Here's how the part is built. I have some questions about the finished solid (model axes, mm). Give positions to 0.01 mm unless a question says otherwise; leave off trailing zeros. Loops run counter-clockwise (first coordinate to the right, second up) from the corner with the lowest first, then second, coordinate; pieces in that order, holes last.
Q1. I need wall thicknesses on line 1 (Z direction, x = -6.5, y = 2.5); line 2 (Z direction, x = -11.5, y = 4.5); line 3 (Z direction, x = 27, y = 2.2). Which ranges of each line are inside material? Lowest first, please.
Q2. If we section it at B-B (z = 39.5): Please give me the cut outline in (x, y), plus the area to 3 significant figures.
Q3. If we section it at C-C (y = 1.4): Give the number of separate pieces and of enclosed holes in the cut face, plus the area to 3 significant figures.
Q4. If we section it at A-A (z = 81): Please give me the cut outline in (x, y), plus the area to 3 significant figures.
Q5. Will these pins go through, and if not, where does the flat tip stop? P1, Ø1.5, axis at y = 2.5, z = -119, coming from the +X side; P2, Ø1.5, axis at x = -4.5, y = 3, coming from the -Z side; P3, Ø8, axis at x = -21, z = 39.5, coming from the +Y side (3 decimals).
from build123d import *

# Parameters (mm, degrees)
BOSS_EXTRUDE1_DEPTH = 5
CHAMFER1_SIZE       = 10
SKETCH2_W           = 52.240142394
SKETCH2_H           = 49.910170897
SKETCH2_H_2         = 19.468376047
CUT_EXTRUDE1_DEPTH  = 5
CHAMFER2_SIZE       = 10


# Some blends are built 0.0001 mm under size
with BuildPart() as part:
    # Sketch1 → Boss-Extrude1 (new body)
    with BuildSketch(Plane(origin=(0, 0, 0), x_dir=(1, 0, 0), z_dir=(0, 1, 0))):
        Polygon((12.5, 112.5), (40, 112.5), (40, -112.5), (-40, -112.5), (-40, 112.5), (-12.5, 112.5), (-12.5, 122.5), (-8, 122.5), (-8, 112.5), (8, 112.5), (8, 122.5), (12.5, 122.5), align=None)
        Polygon((35, -71.386750493), (35, -77.596695784), (35.5, -77.596695784), (35.5, -90.016586366), (-35.5, -90.016586366), (-35.5, -77.596695784), (-35, -77.596695784), (-35, -71.386750493), align=None, mode=Mode.SUBTRACT)
    extrude(amount=BOSS_EXTRUDE1_DEPTH)

    # Chamfer1
    chamfer1_edges = [part.edges().sort_by_distance(p)[0] for p in [
        (-12.5, 2.5, -112.5),
        (12.5, 2.5, -112.5),
    ]]
    chamfer(chamfer1_edges, length=CHAMFER1_SIZE - 0.0001)  # a hair under: the kernel refuses the full size

    # Sketch2 → Cut-Extrude1 (cut)
    with BuildSketch(Plane(origin=(0, 5, 0), x_dir=(1, 0, 0), z_dir=(0, 1, 0))):
        with Locations((0, 36.827678023)):
            Rectangle(SKETCH2_W, SKETCH2_H)
        with Locations((0, -36.827678023)):
            Rectangle(SKETCH2_W, SKETCH2_H)
        with Locations((0, 81.251139518)):
            Rectangle(SKETCH2_W, SKETCH2_H_2)
    extrude(amount=-CUT_EXTRUDE1_DEPTH, mode=Mode.SUBTRACT)

    # Chamfer2
    # the kernel refuses this chamfer: 10 mm, written as the material it adds along each edge
    with BuildSketch(Plane(origin=(26.120071197, 5, -90.985327541), x_dir=(-0.9996219169112968, 0, -0.027495876610586317), z_dir=(0, -1, 0)), Plane(origin=(26.120071197, 5, -71.516951494), x_dir=(0.027495876610586317, 0, -0.9996219169112968), z_dir=(0, -1, 0)), Plane(origin=(-26.120071197, 5, -71.516951494), x_dir=(0.9996219169112968, 0, 0.027495876610586317), z_dir=(0, -1, 0)), Plane(origin=(-26.120071197, 5, 11.872592574), x_dir=(-0.027495876610586667, 0, 0.9996219169112968), z_dir=(0, -1, 0)), Plane(origin=(26.120071197, 5, 11.872592574), x_dir=(-0.9996219169112968, 0, -0.027495876610586317), z_dir=(0, -1, 0)), Plane(origin=(26.120071197, 5, 61.782763471), x_dir=(0.027495876610586317, 0, -0.9996219169112968), z_dir=(0, -1, 0)), Plane(origin=(26.120071197, 5, -61.782763471), x_dir=(-0.9996219169112968, 0, -0.027495876610586317), z_dir=(0, -1, 0)), Plane(origin=(26.120071197, 5, -11.872592574), x_dir=(0.027495876610586324, 0, -0.9996219169112968), z_dir=(0, -1, 0)), Plane(origin=(-26.120071197, 5, -61.782763471), x_dir=(-0.027495876610585973, 0, 0.9996219169112968), z_dir=(0, -1, 0))) as chamfer2_piece_1:
        Polygon((CHAMFER2_SIZE * 0.999621916911, -CHAMFER2_SIZE * 0.0274958766106), (-CHAMFER2_SIZE * 0.0274958766106, -CHAMFER2_SIZE * 0.999621916911), (0, 0), align=None)
    extrude(amount=5)
    with BuildSketch(Plane(origin=(-26.120071197, 5, -90.985327541), x_dir=(0.9996219169112968, 0, -0.027495876610586317), z_dir=(0, -1, 0)), Plane(origin=(-26.120071197, 5, 61.782763471), x_dir=(-0.027495876610585973, 0, -0.9996219169112968), z_dir=(0, -1, 0)), Plane(origin=(-26.120071197, 5, -11.872592574), x_dir=(-0.027495876610586667, 0, -0.9996219169112968), z_dir=(0, -1, 0))) as chamfer2_piece_2:
        Polygon((CHAMFER2_SIZE * 0.999621916911, CHAMFER2_SIZE * 0.0274958766106), (-CHAMFER2_SIZE * 0.0274958766106, CHAMFER2_SIZE * 0.999621916911), (0, 0), align=None)
    extrude(amount=5)


solid = part.part
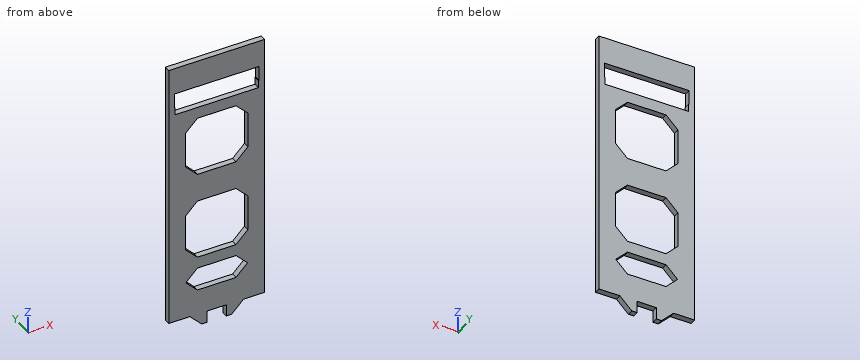
Check sheet entries:
1. line 1: z = -112.5 to -90.99, -71.52 to -61.78, -11.87 to 11.87, 61.78 to 71.39, 90.02 to 112.5
1. line 2: z = -122.5 to -90.99, -71.52 to -61.78, -11.87 to 11.87, 61.78 to 71.39, 90.02 to 112.5
1. line 3: z = -112.5 to 71.39, 90.02 to 112.5
2. outline: (-40, 0) - (-26.12, 0) - (-26.12, 5) - (-40, 5) - close; (26.12, 0) - (40, 0) - (40, 5) - (26.12, 5) - close
2. area: 139 mm2
3. separate pieces: 1
3. enclosed holes: 4
3. area: 11,200 mm2
4. outline: (-40, 0) - (-35.5, 0) - (-35.5, 5) - (-40, 5) - close; (35.5, 0) - (40, 0) - (40, 5) - (35.5, 5) - close
4. area: 45.0 mm2
5. P1: stops at x = 16.75
5. P2: stops at z = -112.5
5. P3: passes through
